```python
from build123d import *

# Parameters (mm, degrees)
F0_W     = 304.8
F0_H     = 171.45
F1_DEPTH = 1.27
F2_W     = 304.8
F2_H     = 2.54
F3_DEPTH = 26.67
F4_W     = 2.54
F4_H     = 171.45
F5_DEPTH = 40.64
F6_R     = 10.16
F7_DEPTH = 304.801


with BuildPart() as f1:
    # F0 (on Front) → F1 (new body, symmetric)
    with BuildSketch(Plane.XZ):
        Rectangle(F0_W, F0_H)
    extrude(amount=F1_DEPTH, both=True)

    # F2 (on face) → F3 (join)
    with BuildSketch(Plane.XZ.offset(1.27)):
        with Locations((0, 84.455)):
            Rectangle(F2_W, F2_H)
    extrude(amount=F3_DEPTH)

    # F4 (on face) → F5 (join)
    with BuildSketch(Plane.XZ.offset(1.27)):
        with Locations((-151.13, 0)):
            Rectangle(F4_W, F4_H)
        with Locations((151.13, 0)):
            Rectangle(F4_W, F4_H)
    extrude(amount=F5_DEPTH)

    # F6 (on face) → F7 (cut, through all)
    with BuildSketch(Plane.YZ.offset(152.4)):
        with Locations((-24.13, 62.865)):
            Circle(F6_R)
        with BuildLine():
            Line((-34.29, -73.025), (-41.91, -73.025))
            Line((-41.91, -73.025), (-41.91, -85.725))
            Line((-41.91, -85.725), (-13.97, -85.725))
            Line((-13.97, -85.725), (-13.97, -61.595))
            ThreePointArc((-13.97, -61.595), (-24.13, -51.435), (-34.29, -61.595))
            Line((-34.29, -61.595), (-34.29, -73.025))
        make_face()
    extrude(amount=-F7_DEPTH, mode=Mode.SUBTRACT)


solid = f1.part
```
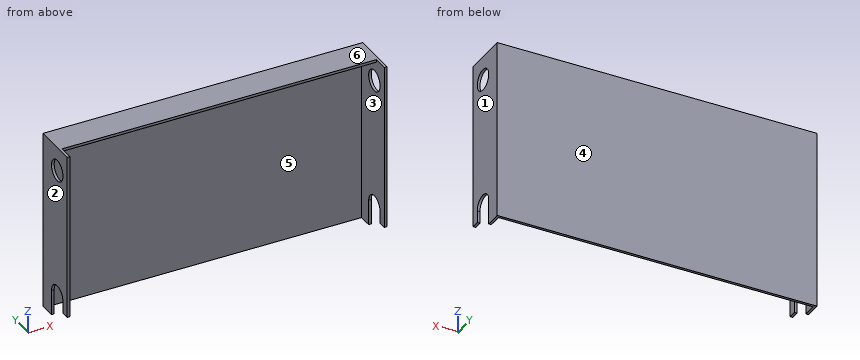
The listing builds one solid part. Answer for the finished solid, in the listing's coordinates (mm). Face numbers are marked on the shaded views. A direction names the side the tool comes from. Round coordinates to 2 decimals unless told otherwise and drop trailing zeros. Write each loop counter-clockwise with the first axis right and the second up, starting at its lowest first coordinate (ties: lowest second). Pieces come first, ordered by that corner, then holes. Notation, with made-up numbers: (-30.5, -26.5) -> (-15.5, -26.5) arc R30 ccw to (-15.5, -0.5) -> close; hole circle Ø2 at (15.5, 55). An arc over 180 degrees is marked (long way). Write item = value, one per line.
1) Section B-B on z = -36 is taken. Write down the section's boundary in (x, y), plus the area to 3 significant figures.
Check values:
outline = (-152.4, -41.91) -> (-149.86, -41.91) -> (-149.86, -1.27) -> (149.86, -1.27) -> (149.86, -41.91) -> (152.4, -41.91) -> (152.4, 1.27) -> (-152.4, 1.27) -> close
area = 981 mm²
2) Section C-C on x = -81 is taken. Write down the section's boundary in (y, z) (3 decimals).
Check values:
outline = (-27.94, 83.185) -> (-1.27, 83.185) -> (-1.27, -85.725) -> (1.27, -85.725) -> (1.27, 85.725) -> (-27.94, 85.725) -> close
3) Section A-A on y = -24.13 is taken. Write down the section's boundary in (x, z) (3 decimals).
Check values:
outline = (-152.4, -51.435) -> (-149.86, -51.435) -> (-149.86, 52.705) -> (-152.4, 52.705) -> close; (-152.4, 73.025) -> (-149.86, 73.025) -> (-149.86, 83.185) -> (149.86, 83.185) -> (149.86, 73.025) -> (152.4, 73.025) -> (152.4, 85.725) -> (-152.4, 85.725) -> close; (149.86, -51.435) -> (152.4, -51.435) -> (152.4, 52.705) -> (149.86, 52.705) -> close
4) Given pin 1 (1.3 mm diameter, centred on x = 151.5, y = -37.5, fed in from -Z) (3 decimals); pin 2 (16.5 mm diameter, centred on y = -24.13, z = 62.865, fed in from +X) (1 decimal); pin 3 (4 mm diameter, centred on x = -31.5, z = -29.5, fed in from -Y); pin 4 (3 mm diameter, centred on x = -27.5, z = 85, fed in from -Y), each flat-ended and moving along its own axis, determine where each tip first touches the part or whether it passes through.
Check values:
pin_1 = -73.025
pin_2 = through
pin_3 = -1.27
pin_4 = -27.94
5) For a pull along X with two mould halves and no side action, classify the marked faces 1, 2, 3 and 4 as released by +X, released by -X, zero draft, split by the parting line, or undercut.
Check values:
face_1 = released by +X
face_2 = released by -X
face_3 = undercut
face_4 = zero draft
6) Which of the six approach directions +Z, -Z, +X, -X, +Y, -Y give full straight-line access (tool end or side, diameter ignored) to the marked faces 5 and 6?
Check values:
face_5 = -Z, -Y
face_6 = +Z, +X, -X, +Y, -Y
7) Straight lines are drawn through the part: line 1 along X through (y, z) = (-19, 77); line 2 along Z through (x, y) = (151, -24) (3 decimals); line 3 along Y through (x, z) = (-125, 71.5). For each, find the intervals that lie inside material, in ascending order. Write a range as [from, to].
Check values:
line_1 = [-152.4, -149.86], [149.86, 152.4]
line_2 = [-51.436, 52.706], [73.024, 85.725]
line_3 = [-1.27, 1.27]
